Check sheet for the modelled part. Datum: model origin and axes. Units: mm. Coordinates: 2 decimals unless noted, no trailing zeros. Write each loop counter-clockwise with the first axis right and the second up, starting at its lowest first coordinate (ties: lowest second). Pieces come first, ordered by that corner, then holes. Notation, with made-up numbers: M 22,-4.5 L 81,-4.5 A28 cw 81,17.5 Z; hole C -33,-27 d7. An arc over 180 degrees is marked long. Answer as CSV lines item,"result". Start each with the question number.
Q1. Thickness scan on line 1 along Z through (x, y) = (31.75, -9) (3 decimals); line 2 along X through (y, z) = (-12.25, 6.35) (3 decimals); line 3 along X through (y, z) = (-10.75, 6.35) (3 decimals). Record the ranges inside material, lowest first. Write a range as from..to.
Q2. Sectioned sample at D-D, the plane x = 50. Record the cut outline in (y, z), then the cut area to 3 significant figures.
Q3. Sectioned sample at B-B, the plane x = 6.35. Record the cut outline in (y, z) (3 decimals), then the cut area to 3 significant figures.
Q4. Sectioned sample at C-C, the plane y = -23. Record the cut outline in (x, z) (3 decimals), then the cut area to 3 significant figures.
Q5. Sectioned sample at A-A, the plane z = 6.35. Record the cut outline in (x, y) (3 decimals), then the cut area to 3 significant figures.
Q6. Depth check by flat-ended pin: pin 1 Ø1 at (y, z) = (-25.5, 5) entering from +X; pin 2 Ø5 at (y, z) = (-22, 5.5) entering from +X; pin 3 Ø1 at (x, z) = (24.5, 3.5) entering from +Y; pin 4 Ø5.5 at (x, z) = (6.35, 6.35) entering from -Y. Enter the tip coordinate at first touch or a pass-through.
Autodesk Inventor part; units mm, degrees
ref_plane "Work Plane1" through (-3.175, 0, 0) normal (1, 0, 0) x (0, 1, 0)
ref_plane "YZ Plane" through (0, 0, 0) normal (1, 0, 0) x (0, 1, 0)
ref_plane "XZ Plane" through (0, 0, 0) normal (0, 1, 0) x (-1, 0, 0)
sketch "Sketch1" plane through (0, 0, 0) normal (0, 0, 1) x (1, 0, 0)
  line L0 (0, 0) -> (38.1, 0)
  line L1 (38.1, 0) -> (56.4309, -31.75)
  line L2 (56.4309, -31.75) -> (-18.3309, -31.75)
  line L3 (-18.3309, -31.75) -> (0, 0)
  dimension "d0" = 38.1
  dimension "d1" = 60
  dimension "d2" = 31.75
extrude "Extrusion1" add sketch "Sketch1" along normal blind 12.7
ref_plane "Work Plane1" through (-3.175, 0, 0) normal (1, 0, 0) x (0, 1, 0)
sketch "Sketch2" plane through (-3.175, 0, 0) normal (1, 0, 0) x (0, 1, 0)
  line L0 (0, 0) -> (0, 12.7)
  circle A0 centre (3.175, 6.35) radius 6.35
  dimension "d5" = 3.175
  dimension "d6" = 12.7
  dimension "d7" = 9.525
extrude "Extrusion2" cut sketch "Sketch2" along normal through all
sketch "Sketch3" plane through (-18.3309, -31.75, 0) normal (0, -1, 0) x (1, 0, 0)
  line L0 (74.7617, 12.7) -> (0, 12.7)
  line L1 (74.7617, 0) -> (0, 0)
  line L2 (74.7617, 0) -> (74.7617, 12.7)
  line L3 (37.3809, 12.7) -> (37.3809, 0) construction
  line L4 (0.4848, 6.35) -> (74.7617, 6.35) construction
  point P0 (24.6809, 6.35)
  point P1 (50.0809, 6.35)
  dimension "d11" = 12.7
  dimension "d12" = 25.4
hole "Hole1" at (6.35, -31.75, 6.35) at (31.75, -31.75, 6.35) direction (0, 1, 0) diameter 6.35 end through all
chamfer "Chamfer1" distance 0.2 angle 45 4 edges at (19.05, -31.75, 12.7) (-18.3309, -31.75, 6.35) (19.05, -31.75, 0) (56.4309, -31.75, 6.35)
properties part number "PWTR-0039" material "Aluminum-6061"
Output:
1,line 1,"z = 0..3.175, 9.525..12.7"
1,line 2,"x = -7.073..3.175, 9.525..28.575, 34.925..45.173"
1,line 3,"x = -6.207..3.175, 9.525..28.575, 34.925..44.307"
2,outline,"M -31.75,0.2 L -31.55,0 L -20.61,0 L -20.61,12.7 L -31.55,12.7 L -31.75,12.5 Z"
2,area,"141 mm^2"
3,outline,"M -31.75,0.2 L -31.55,0 L 0,0 L 0,0.851 A6.35 cw -2.324,3.175 L -31.75,3.175 Z; M -31.75,9.525 L -2.324,9.525 A6.35 cw 0,11.849 L 0,12.7 L -31.55,12.7 L -31.75,12.5 Z"
3,area,"195 mm^2"
4,outline,"M -13.279,0 L 51.379,0 L 51.379,12.7 L -13.279,12.7 Z; hole C 6.35,6.35 d6.35; hole C 31.75,6.35 d6.35"
4,area,"758 mm^2"
5,outline,"M -18.231,-31.577 L -18.131,-31.75 L 3.175,-31.75 L 3.175,-3.175 L -1.833,-3.175 Z; M 9.525,-31.75 L 28.575,-31.75 L 28.575,-3.175 L 9.525,-3.175 Z; M 34.925,-31.75 L 56.231,-31.75 L 56.331,-31.577 L 39.933,-3.175 L 34.925,-3.175 Z"
5,area,"1,300 mm^2"
6,pin 1,"stops at x = 53.11"
6,pin 2,"stops at x = 52.25"
6,pin 3,"stops at y = -2.22"
6,pin 4,"passes through"
